Autodesk Inventor part; units mm, degrees
ref_plane "YZ Plane" through (0, 0, 0) normal (1, 0, 0) x (0, 1, 0)
ref_plane "XZ Plane" through (0, 0, 0) normal (0, 1, 0) x (-1, 0, 0)
ref_plane "XY Plane" through (0, 0, 0) normal (0, 0, 1) x (1, 0, 0)
sketch "スケッチ1" plane through (0, 0, 0) normal (0, 1, 0) x (-1, 0, 0)
  line L0 (4.9789, 14.724) -> (-26.0211, 14.724)
  line L1 (-26.0211, 14.724) -> (-26.0211, -55.276)
  line L2 (-26.0211, -55.276) -> (4.9789, -55.276)
  line L3 (4.9789, -55.276) -> (4.9789, 14.724)
  point P0 (0, 0)
  dimension "d0" = 31
  dimension "d1" = 70
extrude "押し出し1" add sketch "スケッチ1" along normal blind 3
sketch "スケッチ2" plane through (0, 3, 0) normal (0, 1, 0) x (1, 0, 0)
  circle A0 centre (4.0211, -10.724) radius 1.7
  circle A1 centre (17.0211, -10.724) radius 1.7
  line L0 (-4.9789, 55.276) -> (-4.9789, -14.724)
  line L1 (26.0211, -14.724) -> (26.0211, 55.276)
  line L2 (-4.9789, -14.724) -> (26.0211, -14.724)
  circle A2 centre (4.0211, 51.276) radius 1.7
  line L3 (26.0211, 55.276) -> (-4.9789, 55.276)
  circle A3 centre (17.0211, 51.276) radius 1.7
  circle A4 centre (10.5211, 20.276) radius 7.15
  point P0 (0, 0)
  dimension "d4" = 3.4
  dimension "d5" = 3.4
  dimension "d6" = 9
  dimension "d7" = 9
  dimension "d8" = 4
  dimension "d9" = 4
  dimension "d10" = 3.4
  dimension "d11" = 9
  dimension "d12" = 4
  dimension "d13" = 3.4
  dimension "d14" = 9
  dimension "d15" = 4
  dimension "d16" = 14.3
  dimension "d17" = 35
  dimension "d18" = 15.5
hole "穴1" at (4.0211, 3, 10.724) at (17.0211, 3, 10.724) at (17.0211, 3, -51.276) at (4.0211, 3, -51.276) direction (0, -1, 0) diameter 3.4 depth 3
sketch "スケッチ3" plane through (0, 3, 0) normal (0, 1, 0) x (1, 0, 0)
  circle A0 centre (10.5211, 20.276) radius 7.15
  line L0 (-4.9789, 55.276) -> (-4.9789, -14.724)
  line L1 (-4.9789, -14.724) -> (26.0211, -14.724)
  point P0 (0, 0)
  dimension "d26" = 14.3
  dimension "d27" = 15.5
  dimension "d28" = 35
extrude "押し出し2" cut sketch "スケッチ3" against normal blind 3
properties part number "came1"
Source: CAD feature listing. Evaluate the final solid. Frame: model axes, mm. Give positions to 0.01 mm unless a question says otherwise; leave off trailing zeros. Order: outer loops, then holes, each group sorted by start corner. A loop starts at its lowest first (then second) coordinate and runs counter-clockwise, first axis right, second up.
(1) Material intervals for line 1 along Z through (x, y) = (10.5, 2.05); line 2 along X through (y, z) = (0.85, 12); line 3 along X through (y, z) = (2.15, -52), sorted ascending.
(2) Pull-direction query (X, two-part tool) for faces 1 (the face through (26.021, 1, -20)), 2 (the face through (16.51, 1.479, -49.655)), 3 (the face through (10, 1, 14.724)); classes: +X half, -X half, draft (parallel to the pull), parting line (faces both ways), or undercut.
(3) Section query A-A (x = 14.5). Return the cut outline in (y, z), plus the area to 3 significant figures.
(4) Contact query for flat-ended pins moving along their axis: P1, Ø11.5, axis at x = 10.52, z = -20.28, coming from the +Y side; P2, Ø5.5, axis at x = 4.02, z = -51.28, coming from the -Y side. Output: stop coordinate, or through.
(5) Section query C-C (y = 0.85). Return the cut outline in (x, z), plus the area to 3 significant figures.
(6) Section query B-B (z = -23). Return the cut outline in (x, y).
Outcome:
1. line 1: z = -55.28 to -27.43, -13.13 to 14.72
1. line 2: x = -4.98 to 2.9, 5.14 to 15.9, 18.14 to 26.02
1. line 3: x = -4.98 to 2.48, 5.56 to 15.48, 18.56 to 26.02
2. face 1: +X half
2. face 2: undercut
2. face 3: draft
3. outline: (0, -55.28) - (3, -55.28) - (3, -26.22) - (0, -26.22) - close; (0, -14.34) - (3, -14.34) - (3, 14.72) - (0, 14.72) - close
3. area: 174 mm2
4. P1: passes through
4. P2: stops at y = 0
5. outline: (-4.98, -55.28) - (26.02, -55.28) - (26.02, 14.72) - (-4.98, 14.72) - close; hole circle Ø3.4 at (4.02, -51.28); hole circle Ø3.4 at (4.02, 10.72); hole circle Ø14.3 at (10.52, -20.28); hole circle Ø3.4 at (17.02, -51.28); hole circle Ø3.4 at (17.02, 10.72)
5. area: 1,970 mm2
6. outline: (-4.98, 0) - (3.91, 0) - (3.91, 3) - (-4.98, 3) - close; (17.13, 0) - (26.02, 0) - (26.02, 3) - (17.13, 3) - close
